Work out the finished part from the listing and answer in its coordinate system (mm). A direction names the side the tool comes from. Give positions to 0.01 mm unless a question says otherwise; leave off trailing zeros. Order: outer loops, then holes, each group sorted by start corner. A loop starts at its lowest first (then second) coordinate and runs counter-clockwise, first axis right, second up. Notation, with made-up numbers: M 75.5,4.25 L 124.5,4.25 A18 cw 124.5,14.25 Z; hole C 72,-19 d3. An arc over 180 degrees is marked long. One line per item, written item: value.
from build123d import *

# Parameters (mm, degrees)
F0_W     = 2000
F0_H     = 1000
F1_DEPTH = 60
F3_DEPTH = 50
F5_DEPTH = 25


with BuildPart() as f1:
    # F0 (on Front) → F1 (new body)
    with BuildSketch(Plane.XZ):
        with Locations((-239.9550452828, 155.4724135878)):
            Rectangle(F0_W, F0_H)
    extrude(amount=F1_DEPTH)

    # F2 (on face) → F3 (cut)
    with BuildSketch(Plane.XZ.offset(60)):
        with BuildLine():
            Line((-496.3808069078, 305.0812527983), (-976.3808069078, 305.0812527983))
            ThreePointArc((-976.3808069078, 305.0812527983), (-1086.3808069078, 195.0812527983), (-976.3808069078, 85.0812527983))
            Line((-976.3808069078, 85.0812527983), (-496.3808069078, 85.0812527983))
            ThreePointArc((-496.3808069078, 85.0812527983), (-386.3808069078, 195.0812527983), (-496.3808069078, 305.0812527983))
        make_face()
        with BuildLine():
            ThreePointArc((-976.3808069078, 125.0812527983), (-1046.3808069078, 195.0812527983), (-976.3808069078, 265.0812527983))
            Line((-976.3808069078, 265.0812527983), (-496.3808069078, 265.0812527983))
            ThreePointArc((-496.3808069078, 265.0812527983), (-426.3808069078, 195.0812527983), (-496.3808069078, 125.0812527983))
            Line((-496.3808069078, 125.0812527983), (-976.3808069078, 125.0812527983))
        make_face(mode=Mode.SUBTRACT)
    extrude(amount=-F3_DEPTH, mode=Mode.SUBTRACT)

    # F4 (on face) → F5 (cut)
    with BuildSketch(Plane.XZ.offset(60)):
        with BuildLine():
            ThreePointArc((-736.8312674929, 305.0812527983), (-673.7257383371, 356.6361970123), (-594.3531990051, 375.0812527983))
            Line((-594.3531990051, 375.0812527983), (48.4061799943, 375.0812527983))
            ThreePointArc((48.4061799943, 375.0812527983), (228.4061799943, 195.0812527983), (48.4061799943, 15.0812527983))
            Line((48.4061799943, 15.0812527983), (-594.3531990051, 15.0812527983))
            ThreePointArc((-594.3531990051, 15.0812527983), (-673.7257383371, 33.5263085842), (-736.8312674929, 85.0812527983))
            Line((-736.8312674929, 85.0812527983), (-851.8410627968, 85.0812527983))
            ThreePointArc((-851.8410627968, 85.0812527983), (-748.6256852105, -38.5851761127), (-594.3531990051, -84.9187472017))
            Line((-594.3531990051, -84.9187472017), (48.4061799943, -84.9187472017))
            ThreePointArc((48.4061799943, -84.9187472017), (328.4061799943, 195.0812527983), (48.4061799943, 475.0812527983))
            Line((48.4061799943, 475.0812527983), (-594.3531990051, 475.0812527983))
            ThreePointArc((-594.3531990051, 475.0812527983), (-748.6256852105, 428.7476817092), (-851.8410627968, 305.0812527983))
            Line((-851.8410627968, 305.0812527983), (-736.8312674929, 305.0812527983))
        make_face()
        with BuildLine():
            ThreePointArc((-736.8312674929, 85.0812527983), (-774.3531990051, 195.0812527983), (-736.8312674929, 305.0812527983))
            Line((-736.8312674929, 305.0812527983), (-851.8410627968, 305.0812527983))
            ThreePointArc((-851.8410627968, 305.0812527983), (-874.3531990051, 195.0812527983), (-851.8410627968, 85.0812527983))
            Line((-851.8410627968, 85.0812527983), (-736.8312674929, 85.0812527983))
        make_face()
    extrude(amount=-F5_DEPTH, mode=Mode.SUBTRACT)


solid = f1.part
(1) Section C-C, the plane z = 408 is taken. Give the vertices of the cut face in (x, y).
Findings:
outline: M -1239.96,-60 L -776.19,-60 L -776.19,-35 L 230.25,-35 L 230.25,-60 L 760.04,-60 L 760.04,0 L -1239.96,0 Z
(2) Which of the six approach directions +Z, -Z, +X, -X, +Y, -Y give full straight-line access (tool end or side, diameter ignored) to faces 4 (the flat face through (-1239.955, -30, 148)), 5 (the cylindrical face through (-386.407, -35.35, 192.662))?
Findings:
face 4: +Z, -Z, -X, +Y, -Y
face 5: -Y
(3) Find the intervals of material crossed by probe 1 along X at (y, z) = (-48, 197.5); probe 2 along X at (y, z) = (-45, 213); probe 3 along X at (y, z) = (-41, 272), in increasing order. Write a range as from..to.
Findings:
probe 1: x = -1239.96..-1086.35, -1046.34..-874.34, -774.34..-426.42, -386.41..228.39, 328.4..760.04
probe 2: x = -1239.96..-1084.91, -1044.05..-873.78, -773.46..-428.71, -387.85..227.51, 327.83..760.04
probe 3: x = -1239.96..-1055.02, -417.75..211.14, 317.63..760.04
(4) Section B-B, the plane x = -209 is taken. Give the vertices of the cut face in (y, z), then the cut area to 3 significant figures.
Findings:
outline: M -60,-344.53 L 0,-344.53 L 0,655.47 L -60,655.47 L -60,475.08 L -35,475.08 L -35,375.08 L -60,375.08 L -60,15.08 L -35,15.08 L -35,-84.92 L -60,-84.92 Z
area: 55,000 mm^2
(5) Section A-A, the plane y = -50 is taken. Give the vertices of the cut face in (x, z), then the cut area to 3 significant figures.
Findings:
outline: M -1239.96,-344.53 L 760.04,-344.53 L 760.04,655.47 L -1239.96,655.47 Z; M -976.38,125.08 L -865.46,125.08 A280 cw -865.46,265.08 L -976.38,265.08 A70 ccw Z; M -760.18,125.08 L -496.38,125.08 A70 ccw -496.38,265.08 L -760.18,265.08 A180 ccw Z; M -736.83,85.08 A180 ccw -594.35,15.08 L 48.41,15.08 A180 ccw 48.41,375.08 L -594.35,375.08 A180 ccw -736.83,305.08 L -496.38,305.08 A110 cw -496.38,85.08 Z; hole M -976.38,85.08 L -851.84,85.08 A280 ccw -594.35,-84.92 L 48.41,-84.92 A280 ccw 48.41,475.08 L -594.35,475.08 A280 ccw -851.84,305.08 L -976.38,305.08 A110 ccw Z
area: 1,670,000 mm^2
(6) Section D-D, the plane x = -453 is taken. Give the vertices of the cut face in (y, z), then the cut area to 3 significant figures.
Findings:
outline: M -60,-344.53 L 0,-344.53 L 0,655.47 L -60,655.47 L -60,475.08 L -35,475.08 L -35,375.08 L -60,375.08 L -60,296.17 L -10,296.17 L -10,250.02 L -60,250.02 L -60,140.14 L -10,140.14 L -10,94 L -60,94 L -60,15.08 L -35,15.08 L -35,-84.92 L -60,-84.92 Z
area: 50,400 mm^2
(7) Determine the mould class of faces 1 (the flat face through (-154, -60, 198)), 2 (the cylindrical face through (-1046.364, -35.35, 193.542)), 3 (the flat face through (-254, -30, -344.528)) for opening direction Z: pulls with the +Z half, pulls with the -Z half, needs draft (parallel to the pull), parting line crosses it, or undercut.
Findings:
face 1: needs draft
face 2: undercut
face 3: pulls with the -Z half
